Could you check a few things on this model? Use its own coordinates, in mm. A direction names the side the tool comes from. Give positions to 0.01 mm unless a question says otherwise; leave off trailing zeros. Write each loop counter-clockwise with the first axis right and the second up, starting at its lowest first coordinate (ties: lowest second). Pieces come first, ordered by that corner, then holes. Notation, with made-up numbers: (-30.75, 48) - (17.25, 48) arc R30 ccw to (17.25, 83) - close; hole circle Ø2 at (41, -18). An arc over 180 degrees is marked (long way). Write item = value, one per line.
from build123d import *

# Parameters (mm, degrees)
BOSS_EXTRUDE1_DEPTH = 45
SKETCH2_W           = 26.006189056
SKETCH2_H           = 20.126135809
BOSS_EXTRUDE2_DEPTH = 10
SKETCH3_R           = 22.920226204
CUT_EXTRUDE1_DEPTH  = 33
FILLET1_R           = 5
FILLET2_R           = 5


with BuildPart() as part:
    # Sketch1 → Boss-Extrude1 (new body)
    with BuildSketch(Plane.XY):
        Polygon((-70.929913968, 31.492881802), (-70.929913968, -4.255794838), (-56.990550477, -94.56927522), (56.990550477, -94.56927522), (70.929913968, -4.255794838), (70.929913968, 31.492881802), align=None)
    extrude(amount=BOSS_EXTRUDE1_DEPTH)

    # Sketch2 → Boss-Extrude2 (add)
    with BuildSketch(Plane(origin=(70.929913968, 0, 0), x_dir=(0, 0, -1), z_dir=(1, 0, 0))):
        with Locations((-22.5, 13.618543481)):
            Rectangle(SKETCH2_W, SKETCH2_H)
    extrude(amount=BOSS_EXTRUDE2_DEPTH)

    # Sketch3 → Cut-Extrude1 (cut)
    with BuildSketch(Plane.XY.offset(35.503094528)):
        with Locations((95.963397028, 25.985714872)):
            Circle(SKETCH3_R)
    extrude(amount=-CUT_EXTRUDE1_DEPTH, mode=Mode.SUBTRACT)

    # Fillet1
    fillet1_edges = [part.edges().sort_by_distance(p)[0] for p in [
        (-63.960232222, -49.412535029, 45),
        (70.929913968, 31.492881802, 22.5),
        (70.929913968, -4.255794838, 22.5),
        (56.990550477, -94.56927522, 22.5),
        (-56.990550477, -94.56927522, 22.5),
        (-70.929913968, -4.255794838, 22.5),
        (-70.929913968, 31.492881802, 22.5),
        (63.960232222, -49.412535029, 45),
        (70.929913968, 13.618543482, 45),
        (0, 31.492881802, 45),
        (70.929913968, 13.618543482, 0),
        (63.960232222, -49.412535029, 0),
        (-70.929913968, 13.618543482, 45),
        (-63.960232222, -49.412535029, 0),
        (-70.929913968, 13.618543482, 0),
        (0, 31.492881802, 0),
    ]]
    fillet(fillet1_edges, radius=FILLET1_R)

    # Fillet2
    # the kernel refuses this fillet: 5 mm, written as the material it takes off along each edge
    with BuildSketch(Plane(origin=(80.929913968, 8.684525424, 4.131557715), x_dir=(0, -1, 0), z_dir=(0, 0, 1))) as fillet2_piece_1:
        with BuildLine():
            CenterArc((2.146139103, -5), FILLET2_R, 90, 44.149416871)
            ThreePointArc((-1.336520459, -1.412370925), (-0.653275696, -0.720365262), (0, 0))
            Line((0, 0), (2.146139103, 0))
        make_face()
    extrude(amount=36.736884569, mode=Mode.SUBTRACT)
    with BuildSketch(Plane(origin=(73.159277304, 23.681611386, 1.019055512), x_dir=(-1, 0, 0), z_dir=(0, 0, 1))) as fillet2_piece_2:
        with BuildLine():
            CenterArc((4.256496735, 4.570637831), FILLET2_R, 194.254416025, 51.827716126)
            ThreePointArc((-0.589562939, 3.339497856), (-0.232935215, 1.680667414), (0, 0))
            Line((0, 0), (2.229363336, 0))
        make_face()
    extrude(amount=42.961888977, mode=Mode.SUBTRACT)
    with BuildSketch(Plane(origin=(95.963397028, 25.985714872, 9.496905472), x_dir=(-0.9027297705617247, 0.43020804425484166, 0), z_dir=(0.43020804425484166, 0.9027297705617247, 0))) as fillet2_piece_3_section:
        with BuildLine():
            CenterArc((22.920226204 + FILLET2_R, FILLET2_R), FILLET2_R, 180, 90)
            Line((22.920226204, FILLET2_R), (22.920226204, 0))
            Line((22.920226204, 0), (22.920226204 + FILLET2_R, 0))
        make_face()
    fillet2_piece_3 = revolve(axis=Axis((95.963397028, 25.985714872, 9.496905472), (0, 0, 1)), revolution_arc=105.742769493, mode=Mode.PRIVATE)
    fillet2_piece_3 = split(fillet2_piece_3, bisect_by=Plane(origin=(70.929913968, 25.985714872, 9.496905472), z_dir=(1, 0, 0)), keep=Keep.TOP, mode=Mode.PRIVATE)
    add(fillet2_piece_3, mode=Mode.SUBTRACT)
    with BuildSketch(Plane(origin=(95.963397028, 25.985714872, 35.503094528), x_dir=(-0.9027297705617229, 0.4302080442548457, 0), z_dir=(0.4302080442548457, 0.9027297705617229, 0))) as fillet2_piece_4_section:
        with BuildLine():
            CenterArc((22.920226204 + FILLET2_R, -FILLET2_R), FILLET2_R, 90, 90)
            Line((22.920226204, -FILLET2_R), (22.920226204, 0))
            Line((22.920226204, 0), (22.920226204 + FILLET2_R, 0))
        make_face()
    fillet2_piece_4 = revolve(axis=Axis((95.963397028, 25.985714872, 35.503094528), (0, 0, 1)), revolution_arc=105.742769493, mode=Mode.PRIVATE)
    fillet2_piece_4 = split(fillet2_piece_4, bisect_by=Plane(origin=(70.929913968, 25.985714872, 35.503094528), z_dir=(1, 0, 0)), keep=Keep.TOP, mode=Mode.PRIVATE)
    add(fillet2_piece_4, mode=Mode.SUBTRACT)


solid = part.part
1. Which directions (+Z, -Z, +X, -X, +Y, -Y) give clear straight access to the entire face, cutting with the end or side of a thin tool? Please do faces 1 (the face through (70.93, 1, 22)), 2 (the face through (73, 6, 9.497)), 3 (the face through (76, 3.555, 23)).
Filled sheet:
face_1 = +X
face_2 = -Z, +X, +Y, -Y
face_3 = +Z, -Z, +X, -Y
2. For pin 1 (1.5 mm diameter, centred on y = -61.5, z = 6, fed in from +X); pin 2 (1.5 mm diameter, centred on y = -17.5, z = 31.5, fed in from +X); pin 3 (24.5 mm diameter, centred on y = 8.5, z = 31, fed in from +X); pin 4 (2 mm diameter, centred on x = -54.5, z = 19, fed in from -Y), each with a flat end and sliding along its axis, tell me the tip position at first contact or that it passes through.
Filled sheet:
pin_1 = 62.21
pin_2 = 69
pin_3 = 80.93
pin_4 = -94.51
3. I need wall thicknesses on line 1 (X direction, y = -4, z = 9.5); line 2 (X direction, y = -62, z = 23.5); line 3 (Y direction, x = -36, z = 3). Which ranges of each line are inside material? Lowest first, please.
Filled sheet:
line_1 = -70.93 to 70.93
line_2 = -62.02 to 62.02
line_3 = -94.57 to 31.08
4. If we section it at A-A, the plane z = 26.5: Please give me the cut outline in (x, y).
Filled sheet:
outline = (-70.93, -3.87) arc R5 ccw to (-70.87, -4.63) - (-57.64, -90.33) arc R5 ccw to (-52.7, -94.57) - (52.7, -94.57) arc R5 ccw to (57.64, -90.33) - (70.87, -4.63) arc R5 ccw to (70.93, -3.87) - (70.93, 3.56) - (80.93, 3.56) - (80.93, 6.54) arc R5 ccw to (79.52, 10.02) arc R22.92 cw to (73.75, 20.34) arc R5 ccw to (70.93, 23.68) - (70.93, 26.49) arc R5 ccw to (65.93, 31.49) - (-65.93, 31.49) arc R5 ccw to (-70.93, 26.49) - close
